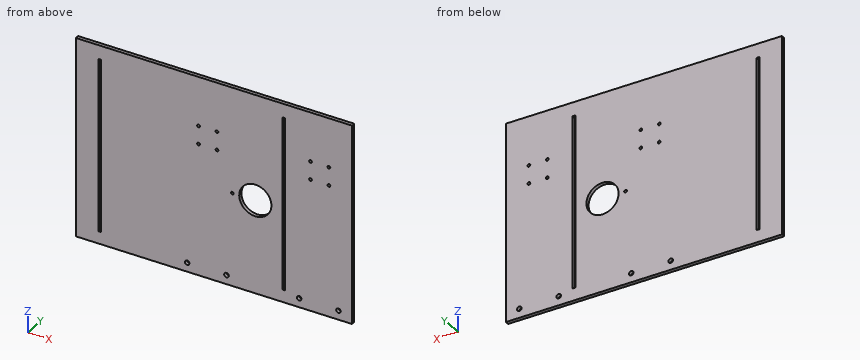
from build123d import *

# Parameters (mm, degrees)
SKETCH1_W               = 300
SKETCH1_H               = 219
SKETCH1_W_2             = 3
SKETCH1_H_2             = 190.1710485
BOSS_EXTRUDE1_DEPTH     = 4
SKETCH2_R               = 17.5
CUT_EXTRUDE2_DEPTH      = 186.758579883
CUT_EXTRUDE3_DEPTH      = 186.758579883
CUT_EXTRUDE3_DEPTH_BACK = 186.758579883
SKETCH3_R               = 1.5
CUT_EXTRUDE4_DEPTH      = 186.758579883
CUT_EXTRUDE4_DEPTH_BACK = 186.758579883
SKETCH4_R               = 1.5
CUT_EXTRUDE5_DEPTH      = 186.758579883
CUT_EXTRUDE5_DEPTH_BACK = 186.758579883
SKETCH5_R               = 2.5
CUT_EXTRUDE6_DEPTH      = 186.758579883
CUT_EXTRUDE6_DEPTH_BACK = 186.758579883
SKETCH6_R               = 2.5
CUT_EXTRUDE7_DEPTH      = 186.758579883
CUT_EXTRUDE7_DEPTH_BACK = 186.758579883
SKETCH7_R               = 1.5


with BuildPart() as part:
    # Sketch1 → Boss-Extrude1 (new body)
    with BuildSketch(Plane(origin=(0, 0, 0), x_dir=(1, 0, 0), z_dir=(0, 1, 0))):
        Rectangle(SKETCH1_W, SKETCH1_H)
        with Locations((-124, 0.80041533)):
            Rectangle(SKETCH1_W_2, SKETCH1_H_2, mode=Mode.SUBTRACT)
        with Locations((76, 0.80041533)):
            Rectangle(SKETCH1_W_2, SKETCH1_H_2, mode=Mode.SUBTRACT)
    extrude(amount=BOSS_EXTRUDE1_DEPTH)

    # Sketch2 → Cut-Extrude2 (cut, through all)
    with BuildSketch(Plane(origin=(0, 0, 0), x_dir=(-1, 0, 0), z_dir=(0, -1, 0))):
        with Locations(Location((-45, 7, 0), (0, 0, 90))):
            Circle(SKETCH2_R)
    extrude(amount=-CUT_EXTRUDE2_DEPTH, mode=Mode.SUBTRACT)

    # Sketch3 → Cut-Extrude3 (cut, two sides: drawn at the far end of the back side and taken through both)
    with BuildSketch(Plane(origin=(0, 0, 0), x_dir=(-1, 0, 0), z_dir=(0, -1, 0)).offset(-CUT_EXTRUDE3_DEPTH_BACK)):
        with Locations(Location((-125, -55.39, 0), (0, 0, 90))):
            Circle(SKETCH3_R)
        with Locations(Location((-125, -35.39, 0), (0, 0, 90))):
            Circle(SKETCH3_R)
        with Locations(Location((-105, -35.39, 0), (0, 0, 90))):
            Circle(SKETCH3_R)
        with Locations(Location((-105, -55.39, 0), (0, 0, 90))):
            Circle(SKETCH3_R)
    extrude(amount=CUT_EXTRUDE3_DEPTH + CUT_EXTRUDE3_DEPTH_BACK, mode=Mode.SUBTRACT)

    # Sketch4 → Cut-Extrude4 (cut, two sides: drawn at the far end of the back side and taken through both)
    with BuildSketch(Plane(origin=(0, 0, 0), x_dir=(-1, 0, 0), z_dir=(0, -1, 0)).offset(-CUT_EXTRUDE4_DEPTH_BACK)):
        with Locations(Location((-3.32, -55.39, 0), (0, 0, 90))):
            Circle(SKETCH4_R)
        with Locations(Location((-3.32, -35.39, 0), (0, 0, 90))):
            Circle(SKETCH4_R)
        with Locations(Location((16.68, -35.39, 0), (0, 0, 90))):
            Circle(SKETCH4_R)
        with Locations(Location((16.68, -55.39, 0), (0, 0, 90))):
            Circle(SKETCH4_R)
    extrude(amount=CUT_EXTRUDE4_DEPTH + CUT_EXTRUDE4_DEPTH_BACK, mode=Mode.SUBTRACT)

    # Sketch5 → Cut-Extrude5 (cut, two sides: drawn at the far end of the back side and taken through both)
    with BuildSketch(Plane(origin=(0, 0, 0), x_dir=(-1, 0, 0), z_dir=(0, -1, 0)).offset(-CUT_EXTRUDE5_DEPTH_BACK)):
        with Locations(Location((-135.39, 99.5, 0), (0, 0, 90))):
            Circle(SKETCH5_R)
        with Locations(Location((-92.61, 99.5, 0), (0, 0, 90))):
            Circle(SKETCH5_R)
    extrude(amount=CUT_EXTRUDE5_DEPTH + CUT_EXTRUDE5_DEPTH_BACK, mode=Mode.SUBTRACT)

    # Sketch6 → Cut-Extrude6 (cut, two sides: drawn at the far end of the back side and taken through both)
    with BuildSketch(Plane.XZ.offset(-CUT_EXTRUDE6_DEPTH_BACK)):
        with Locations(Location((13.71, -99.5, 0), (0, 0, 270))):
            Circle(SKETCH6_R)
        with Locations(Location((-29.07, -99.5, 0), (0, 0, 270))):
            Circle(SKETCH6_R)
    extrude(amount=CUT_EXTRUDE6_DEPTH + CUT_EXTRUDE6_DEPTH_BACK, mode=Mode.SUBTRACT)

    # Sketch7 → Cut-Extrude7 (cut, two sides: drawn at the far end of the back side and taken through both)
    with BuildSketch(Plane(origin=(0, 4, 0), x_dir=(1, 0, 0), z_dir=(0, 1, 0)).offset(-CUT_EXTRUDE7_DEPTH_BACK)):
        with Locations(Location((20, 7, 0), (0, 0, 270))):
            Circle(SKETCH7_R)
    extrude(amount=CUT_EXTRUDE7_DEPTH + CUT_EXTRUDE7_DEPTH_BACK, mode=Mode.SUBTRACT)


solid = part.part
Geometry: final body of the model. Coordinates: model frame, mm. Round coordinates to 2 decimals unless told otherwise and drop trailing zeros. Order: outer loops, then holes, each group sorted by start corner. A loop starts at its lowest first (then second) coordinate and runs counter-clockwise, first axis right, second up.
Q1. Section A-A, the plane z = 40. Output: boundary loops of the cut face in (x, y).
Result sheet:
outline: (-150, 0) - (-125.5, 0) - (-125.5, 4) - (-150, 4) - close; (-122.5, 0) - (74.5, 0) - (74.5, 4) - (-122.5, 4) - close; (77.5, 0) - (150, 0) - (150, 4) - (77.5, 4) - close
Q2. Section B-B, the plane y = 3.2. Give the number of separate pieces and of enclosed holes in the cut face, and give its area (3 significant figures).
Result sheet:
separate pieces: 1
enclosed holes: 16
area: 63,500 mm2
Q3. Section C-C, the plane x = 35. Output: boundary loops of the cut face in (y, z).
Result sheet:
outline: (0, -109.5) - (4, -109.5) - (4, -21.36) - (0, -21.36) - close; (0, 7.36) - (4, 7.36) - (4, 109.5) - (0, 109.5) - close
Q4. Material intervals for probe 1 along X at (y, z) = (2.45, -99.5); probe 2 along X at (y, z) = (1, -45); probe 3 along X at (y, z) = (3, -7), sorted ascending.
Result sheet:
probe 1: x = -150 to -31.57, -26.57 to 11.21, 16.21 to 90.11, 95.11 to 132.89, 137.89 to 150
probe 2: x = -150 to -125.5, -122.5 to 74.5, 77.5 to 150
probe 3: x = -150 to -125.5, -122.5 to 18.5, 21.5 to 27.5, 62.5 to 74.5, 77.5 to 150
Q5. Pin query (flat end, axial travel): pin 1 (1.8 mm diameter, centred on x = 3.32, z = 35.39, fed in from -Y). Return the tip coordinate at first contact, or that it passes through.
Result sheet:
pin 1: passes through
